Verification items for the finished model (mm, model axes). A direction names the side the tool comes from. Coordinates: 2 decimals unless noted, no trailing zeros. Write each loop counter-clockwise with the first axis right and the second up, starting at its lowest first coordinate (ties: lowest second). Pieces come first, ordered by that corner, then holes. Notation, with made-up numbers: (30, 76.25) -> (43, 76.25) arc R33 cw to (43, 109.25) -> close; hole circle Ø11 at (81, 41). An arc over 180 degrees is marked (long way). Answer in a Markdown table with one row per item.
Autodesk Inventor part; units mm, degrees
ref_plane "YZ Plane" through (0, 0, 0) normal (1, 0, 0) x (0, 1, 0)
ref_plane "XZ Plane" through (0, 0, 0) normal (0, 1, 0) x (-1, 0, 0)
ref_plane "XY Plane" through (0, 0, 0) normal (0, 0, 1) x (1, 0, 0)
sketch "Boceto1" plane through (0, 0, 0) normal (0, 1, 0) x (-1, 0, 0)
  line L0 (-40, 8) -> (40, 8)
  line L1 (40, 8) -> (40, -8)
  line L2 (40, -8) -> (-40, -8)
  line L3 (-40, -8) -> (-40, 8)
  line L4 (-40, 8) -> (40, -8) construction
  line L5 (40, 8) -> (-40, -8) construction
  circle A0 centre (-34, 4) radius 2.7
  circle A1 centre (-34, -4) radius 2.7
  circle A2 centre (16.7, 4) radius 2.7
  circle A3 centre (16.7, -4) radius 2.7
  line L6 (19.4, 4) -> (14, 4)
  line L7 (14, 4) -> (14, -4)
  line L8 (14, -4) -> (19.4, -4)
  line L9 (19.4, -4) -> (19.4, 4)
  line L10 (-31.3, 4) -> (-36.7, 4)
  line L11 (-36.7, 4) -> (-36.7, -4)
  line L12 (-36.7, -4) -> (-31.3, -4)
  line L13 (-31.3, -4) -> (-31.3, 4)
  point P0 (0, 0)
  point P1 (16.7, -4)
  point P2 (16.7, 4)
  point P3 (-34, -4)
  point P4 (-34, 4)
  point P5 (19.4, -4)
  point P6 (-31.3, -4)
  dimension "d2" = 5.4
  dimension "d0" = 80
  dimension "d1" = 16
  dimension "d3" = 4
  dimension "d4" = 8
  dimension "d5" = 6
  dimension "d6" = 50.7
extrude "Extrusión1" add sketch "Boceto1" along normal blind 5
sketch "Boceto2" plane through (0, 5, 0) normal (0, 1, 0) x (1, 0, 0)
  circle A0 centre (20, 4.1) radius 3.9
  circle A1 centre (-30, 4.1) radius 3.9
  line L0 (40, 8) -> (-40, 8)
  line L1 (40, -8) -> (40, 8)
  line L2 (-40, 8) -> (-40, -8)
  point P0 (0, 0)
  dimension "d11" = 7.8
  dimension "d12" = 20
  dimension "d13" = 10
extrude "Extrusión2" add sketch "Boceto2" along normal blind 13
sketch "Boceto3" plane through (0, 5, 0) normal (0, 1, 0) x (1, 0, 0)
  line L0 (31.3, -4) -> (31.3, 4)
  arc A0 (36.7, 4) -> (31.3, 4) centre (34, 4) ccw
  line L1 (36.7, 4) -> (36.7, -4)
  arc A1 (31.3, -4) -> (36.7, -4) centre (34, -4) ccw
  line L2 (-19.4, -4) -> (-19.4, 4)
  arc A2 (-14, 4) -> (-19.4, 4) centre (-16.7, 4) ccw
  line L3 (-14, 4) -> (-14, -4)
  arc A3 (-19.4, -4) -> (-14, -4) centre (-16.7, -4) ccw
  line L4 (40, 8) -> (20, 8)
  circle A4 centre (20, 4.1) radius 3.9
  line L5 (20, 8) -> (-30, 8)
  circle A5 centre (-30, 4.1) radius 3.9
  line L6 (-30, 8) -> (-40, 8)
  line L7 (-40, 8) -> (-40, -8)
  line L8 (-40, -8) -> (40, -8)
  line L9 (40, -8) -> (40, 8)
  circle A6 centre (-30, 4.1) radius 3.9
  circle A7 centre (-30, 4.1) radius 6
  circle A8 centre (20, 4.1) radius 3.9
  circle A9 centre (20, 4.1) radius 6
  point P0 (0, 0)
  point P1 (15.4404, 8)
  point P2 (24.5596, 8)
  point P3 (-34.5596, 8)
  point P4 (-25.4404, 8)
  dimension "d14" = 12
  dimension "d15" = 12
extrude "Extrusión3" add sketch "Boceto3" along normal blind 8 contours A9 L5 L4 | A7 L6 L5 picked at (25.2424, 3.6235) picked at (-24.7576, 3.6235)
fillet "Empalme1" radius 2 2 edges at (20, 5, 1.9) (-30, 5, 1.9)
sketch "Boceto4" plane through (-30, 18, -4.1) normal (0, 1, 0) x (1, 0, 0)
  circle A0 centre (0, 0) radius 3.9
  circle A1 centre (0, 0) radius 1.7
  circle A2 centre (50, 0) radius 3.9
  circle A3 centre (50, 0) radius 1.7
  point P0 (30, -4.1)
  dimension "d19" = 3.4
  dimension "d20" = 3.4
extrude "Extrusión4" cut sketch "Boceto4" against normal through all contours A1 | A3
fillet "Empalme2" radius 3 4 edges at (-40, 2.5, 8) (-40, 2.5, -8) (40, 2.5, 8) (40, 2.5, -8)
sketch "Boceto5" plane through (0, 0, 0) normal (0, -1, 0) x (1, 0, 0)
  circle A0 centre (-30, -4.1) radius 1.7
  circle A1 centre (-30, -4.1) radius 2.875
  circle A2 centre (20, -4.1) radius 1.7
  circle A3 centre (20, -4.1) radius 2.875
  line L0 (-33.3198, -4.1) -> (-31.6599, -1.225)
  line L1 (-31.6599, -1.225) -> (-28.3401, -1.225)
  line L2 (-28.3401, -1.225) -> (-26.6802, -4.1)
  line L3 (-26.6802, -4.1) -> (-28.3401, -6.975)
  line L4 (-28.3401, -6.975) -> (-31.6599, -6.975)
  line L5 (-31.6599, -6.975) -> (-33.3198, -4.1)
  line L6 (16.6802, -4.1) -> (18.3401, -1.225)
  line L7 (18.3401, -1.225) -> (21.6599, -1.225)
  line L8 (21.6599, -1.225) -> (23.3198, -4.1)
  line L9 (23.3198, -4.1) -> (21.6599, -6.975)
  line L10 (21.6599, -6.975) -> (18.3401, -6.975)
  line L11 (18.3401, -6.975) -> (16.6802, -4.1)
  point P0 (0, 0)
  dimension "d24" = 5.75
extrude "Extrusión5" cut sketch "Boceto5" against normal blind 5.5 contours A0 | A1 | A1 L2 L3 | A1 L1 L2 | L3 L4 A1 | A1 L0 L1 | L4 L5 A1 | A1 L5 L0 | A2 | A3 | A3 L8 L9 | A3 L7 L8 | L9 L10 A3 | A3 L6 L7 | L10 L11 A3 | A3 L11 L6
properties part number "Rack support"
1. Section check C-C, the plane y = 16. Record the boundary of the cut face in (x, z).
Geometry says:
| item | result |
|---|---|
| outline | circle Ø7.8 at (-30, -4.1); circle Ø7.8 at (20, -4.1); hole circle Ø3.4 at (-30, -4.1); hole circle Ø3.4 at (20, -4.1) |
2. Tool access check on faces 5 (the flat face through (-28, 18, -3)), 6 (the cylindrical face through (-39.14, 2.54, 7.1)), 7 (the flat face through (22.5, 2.71, -5.52)), 8 (the flat face through (31.3, 2, 0)), 9 (the cylindrical face through (-29.809, 9.958, 1.897)). Record the directions out of +Z, -Z, +X, -X, +Y, -Y that give a thin tool (end or side, any length) a straight path to the whole face; none if there is none.
Geometry says:
| item | result |
|---|---|
| face 5 | +Z, -Z, +X, -X, +Y |
| face 6 | +Z, -X, +Y, -Y |
| face 7 | -Y |
| face 8 | +Y, -Y |
| face 9 | +Y |
3. Thickness scan on line 1 (X direction, y = 14.5, z = -4.1); line 2 (X direction, y = 9.5, z = -4.1); line 3 (X direction, y = 3.5, z = 3). Record the ranges inside material, lowest first. Write a range as from..to.
Geometry says:
| item | result |
|---|---|
| line 1 | -33.9..-31.7, -28.3..-26.1, 16.1..18.3, 21.7..23.9 |
| line 2 | -36..-31.7, -28.3..-24, 14..18.3, 21.7..26 |
| line 3 | -40..-19.4, -14..31.3, 36.7..40 |
4. Section check B-B, the plane y = 2.5. Record the boundary of the cut face in (x, z) (3 decimals), plus the area to 3 significant figures.
Geometry says:
| item | result |
|---|---|
| outline | (-40, -5) arc R3 ccw to (-37, -8) -> (37, -8) arc R3 ccw to (40, -5) -> (40, 5) arc R3 ccw to (37, 8) -> (-37, 8) arc R3 ccw to (-40, 5) -> close; hole (-33.32, -4.1) -> (-31.66, -6.975) -> (-28.34, -6.975) -> (-26.68, -4.1) -> (-28.34, -1.225) -> (-31.66, -1.225) -> close; hole (-19.4, -4) arc R2.7 ccw to (-14, -4) -> (-14, 4) arc R2.7 ccw to (-19.4, 4) -> close; hole (16.68, -4.1) -> (18.34, -6.975) -> (21.66, -6.975) -> (23.32, -4.1) -> (21.66, -1.225) -> (18.34, -1.225) -> close; hole (31.3, -4) arc R2.7 ccw to (36.7, -4) -> (36.7, 4) arc R2.7 ccw to (31.3, 4) -> close |
| area | 1,080 mm^2 |
5. Section check D-D, the plane y = 11.25. Record the boundary of the cut face in (x, z), plus the area to 3 significant figures.
Geometry says:
| item | result |
|---|---|
| outline | (-34.56, -8) -> (-25.44, -8) arc R6 ccw (long way) to start; (15.44, -8) -> (24.56, -8) arc R6 ccw (long way) to start; hole circle Ø3.4 at (-30, -4.1); hole circle Ø3.4 at (20, -4.1) |
| area | 181 mm^2 |
6. Section check A-A, the plane x = -16.7. Record the boundary of the cut face in (y, z).
Geometry says:
| item | result |
|---|---|
| outline | (0, -8) -> (5, -8) -> (5, -6.7) -> (0, -6.7) -> close; (0, 6.7) -> (5, 6.7) -> (5, 8) -> (0, 8) -> close |
7. Mould release check, pull along X, two halves, no side actions. Record for faces 1 (the flat face through (40, 2, 0)), 2 (the flat face through (-32.478, 2.712, -5.558)), 3 (the flat face through (1, 0, 0)), 4 (the flat face through (-40, 2, 0)): released by +X, released by -X, zero draft, split by the parting line, or undercut.
Geometry says:
| item | result |
|---|---|
| face 1 | released by +X |
| face 2 | undercut |
| face 3 | zero draft |
| face 4 | released by -X |
8. Depth check by flat-ended pin: P1, Ø6, axis at y = 14, z = -3, coming from the -X side; P2, Ø5.5, axis at x = -30, z = -4.1, coming from the -Y side; P3, Ø8, axis at x = -18, y = 15, coming from the +Z side; P4, Ø5, axis at x = -23, y = 12, coming from the +Z side. Enter the tip coordinate at first touch or a pass-through.
Geometry says:
| item | result |
|---|---|
| P1 | x = -36 |
| P2 | y = 5.5 |
| P3 | through |
| P4 | z = -0.13 |
